Could you check a few things on this model? Use its own coordinates, in mm. Give positions to 0.01 mm unless a question says otherwise; leave off trailing zeros. Order: outer loops, then holes, each group sorted by start corner. A loop starts at its lowest first (then second) coordinate and runs counter-clockwise, first axis right, second up. Notation, with made-up numbers: M 2.5,-14.75 L 42.5,-14.75 A35 cw 42.5,18.25 Z; hole C -27,-23 d8. An arc over 180 degrees is marked long. Use a Markdown table: item, result. Add a question column.
Item 1: If I drill on L1, parallel to Z at x = 44.45, y = -1.15 (3 decimals); L2, parallel to X at y = -2.4, z = 190.5 (3 decimals); L3, parallel to X at y = -1.95, z = 98.5, over which ranges is the centre line in solid material (lowest first)? Write a range as from..to.
Item 2: Suppose I cut it at A-A on x = 14. Write out the boundary of the cut face in (y, z).
Item 3: Suppose I cut it at B-B on y = -1.1. Count the separate pieces of the cut face and the enclosed holes in it, plus the area to 3 significant figures.
Item 4: I'm going to push flat-ended pins straight in: pin 1 Ø5 at (x, z) = (0, 0) entering from +Y; pin 2 Ø1 at (y, z) = (-1, 141) entering from +X; pin 3 Ø1.5 at (y, z) = (-2, 25) entering from -X; pin 4 Ø1.5 at (y, z) = (-2.5, 168) entering from -X. Where does each tip first touch, or does it pass through?
from build123d import *

# Parameters (mm, degrees)
F0_R     = 3.175
F1_DEPTH = 3.048


with BuildPart() as f1:
    # F0 (on Front) → F1 (new body)
    with BuildSketch(Plane.XZ):
        with BuildLine():
            Line((-9.513086, 190.97625), (-15.855144, 64.29375))
            ThreePointArc((-15.855144, 64.29375), (0, 79.375), (15.855144, 64.29375))
            Line((15.855144, 64.29375), (9.513086, 190.97625))
            ThreePointArc((9.513086, 190.97625), (9.522021, 190.738199), (9.525, 190.5))
            ThreePointArc((9.525, 190.5), (-0.238199, 180.977979), (-9.513086, 190.97625))
        make_face()
        with Locations((-3.175, 100.0252)):
            Circle(F0_R, mode=Mode.SUBTRACT)
        with BuildLine():
            ThreePointArc((-9.477255, -0.9525), (-0.476848, 9.513056), (9.525, 0))
            ThreePointArc((9.525, 0), (6.970557, -6.491299), (0.677344, -9.500886))
            Line((0.677344, -9.500886), (44.732405, -7.932475))
            ThreePointArc((44.732405, -7.932475), (36.5125, 0.000539), (44.733482, 7.932436))
            Line((44.733482, 7.932436), (18.9676, 8.853234))
            ThreePointArc((18.9676, 8.853234), (13.2612, 11.571359), (11.341187, 17.593382))
            Line((11.341187, 17.593382), (15.795426, 61.9125))
            ThreePointArc((15.795426, 61.9125), (0, 47.625), (-15.795426, 61.9125))
            Line((-15.795426, 61.9125), (-9.477255, -0.9525))
        make_face()
        with BuildLine():
            ThreePointArc((-15.855144, 64.29375), (-15.87001, 63.102003), (-15.795426, 61.9125))
            ThreePointArc((-15.795426, 61.9125), (0, 47.625), (15.795426, 61.9125))
            ThreePointArc((15.795426, 61.9125), (15.855094, 62.705253), (15.875, 63.5))
            ThreePointArc((15.875, 63.5), (15.870035, 63.896999), (15.855144, 64.29375))
            ThreePointArc((15.855144, 64.29375), (0, 79.375), (-15.855144, 64.29375))
        make_face()
        with Locations((0, 63.5)):
            Circle(F0_R, mode=Mode.SUBTRACT)
        with BuildLine():
            ThreePointArc((0.677344, -9.500886), (6.970557, -6.491299), (9.525, 0))
            ThreePointArc((9.525, 0), (-0.476848, 9.513056), (-9.477255, -0.9525))
            ThreePointArc((-9.477255, -0.9525), (-6.389564, -7.063929), (0, -9.525))
            Line((0, -9.525), (0.677344, -9.500886))
        make_face()
        Circle(F0_R, mode=Mode.SUBTRACT)
        with BuildLine():
            ThreePointArc((44.733482, 7.932436), (36.5125, 0.000539), (44.732405, -7.932475))
            ThreePointArc((44.732405, -7.932475), (50.161633, -5.51191), (52.3875, 0))
            ThreePointArc((52.3875, 0), (50.162007, 5.511523), (44.733482, 7.932436))
        make_face()
        with Locations((44.45, 0)):
            Circle(F0_R, mode=Mode.SUBTRACT)
        with BuildLine():
            ThreePointArc((9.513086, 190.97625), (0, 200.025), (-9.513086, 190.97625))
            ThreePointArc((-9.513086, 190.97625), (-0.238199, 180.977979), (9.525, 190.5))
            ThreePointArc((9.525, 190.5), (9.522021, 190.738199), (9.513086, 190.97625))
        make_face()
        with Locations((0, 190.5)):
            Circle(F0_R, mode=Mode.SUBTRACT)
    extrude(amount=F1_DEPTH)


solid = f1.part
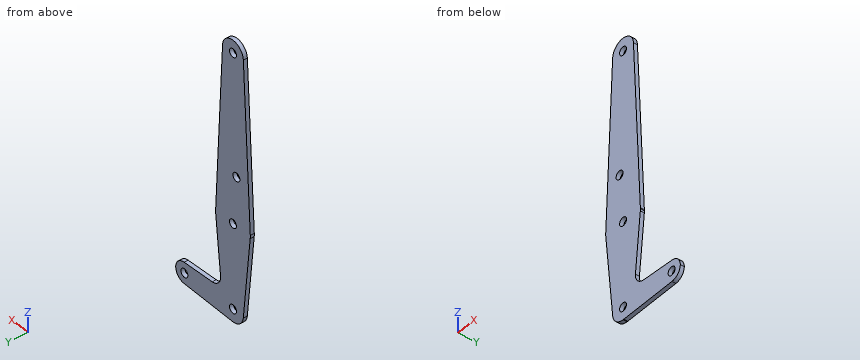
Findings below:
| question | item | result |
|---|---|---|
| 1 | L1 | z = -7.943..-3.175, 3.175..7.943 |
| 1 | L2 | x = -9.537..-3.175, 3.175..9.537 |
| 1 | L3 | x = -14.14..-5.96, -0.39..14.14 |
| 2 | outline | M -3.05,-9.03 L 0,-9.03 L 0,10.83 L -3.05,10.83 Z; M -3.05,44.05 L 0,44.05 L 0,101.35 L -3.05,101.35 Z |
| 3 | separate pieces | 1 |
| 3 | enclosed holes | 5 |
| 3 | area | 5,700 mm^2 |
| 4 | pin 1 | passes through |
| 4 | pin 2 | stops at x = 12.04 |
| 4 | pin 3 | stops at x = -12.16 |
| 4 | pin 4 | stops at x = -10.7 |
